from build123d import *

# Parameters (mm, degrees)
BOSS_EXTRUDE1_DEPTH = 5.0165
SKETCH2_W           = 41.021
SKETCH2_H           = 23.876
BOSS_EXTRUDE2_DEPTH = 11.049


with BuildPart() as part:
    # Sketch1 → Boss-Extrude1 (new, symmetric)
    with BuildSketch(Plane(origin=(0, 0, 0), x_dir=(1, 0, 0), z_dir=(0, 1, 0))):
        Polygon((-18.8595, 0), (18.8595, 0), (20.4978, 6.6675), (27.3558, 6.6675), (27.3558, 10.0838), (44.5897, 10.0838), (44.5897, 0.9398), (49.1871, 0.9398), (49.1871, -5.1943), (39.497, -5.1943), (39.497, -18.4404), (-39.497, -18.4404), (-39.497, -5.1943), (-49.1871, -5.1943), (-49.1871, 0.9398), (-44.5897, 0.9398), (-44.5897, 10.0838), (-27.3558, 10.0838), (-27.3558, 6.6675), (-20.4978, 6.6675), align=None)
    extrude(amount=BOSS_EXTRUDE1_DEPTH, both=True)

    # Sketch2 → Boss-Extrude2 (add, symmetric)
    with BuildSketch(Plane(origin=(0, 0, 0), x_dir=(1, 0, 0), z_dir=(0, 1, 0))):
        with Locations((0, -30.3784)):
            Rectangle(SKETCH2_W, SKETCH2_H)
    extrude(amount=BOSS_EXTRUDE2_DEPTH, both=True)


solid = part.part
Can you work these out from the model? Positions are in its coordinate system, mm. A direction names the side the tool comes from. Coordinates: 2 decimals unless noted, no trailing zeros. Write each loop counter-clockwise with the first axis right and the second up, starting at its lowest first coordinate (ties: lowest second). Pieces come first, ordered by that corner, then holes. Notation, with made-up numbers: M 27.25,12 L 63.25,12 A29 cw 63.25,36 Z; hole C 77,-31.75 d8. An arc over 180 degrees is marked long. Use one line per item in the form item = value.
Q1. For faces 1 (the flat face through (0, 0, 0)), 2 (the flat face through (-44.59, 0, -5)), 3 (the flat face through (20.51, 0, 31)), which set-ups out of +Z, -Z, +X, -X, +Y, -Y let a thin tool reach every point of the face, with its end or its side?
Model answer:
face_1 = -Z, +Y, -Y
face_2 = -Z, -X, +Y, -Y
face_3 = +Z, +X, +Y, -Y
Q2. If we section it at B-B (z = -3.5): Write out the boundary of the cut face in (x, y).
Model answer:
outline = M -44.59,-5.02 L -19.72,-5.02 L -19.72,5.02 L -44.59,5.02 Z; M 19.72,-5.02 L 44.59,-5.02 L 44.59,5.02 L 19.72,5.02 Z
Q3. If we section it at D-D (z = 9.5): Write out the boundary of the cut face in (x, y), then the cut area to 3 significant figures.
Model answer:
outline = M -39.5,-5.02 L 39.5,-5.02 L 39.5,5.02 L -39.5,5.02 Z
area = 793 mm^2
Q4. If we section it at C-C (y = -1.75): Write out the boundary of the cut face in (x, z), then the cut area to 3 significant figures.
Model answer:
outline = M -49.19,-0.94 L -44.59,-0.94 L -44.59,-10.08 L -27.36,-10.08 L -27.36,-6.67 L -20.5,-6.67 L -18.86,0 L 18.86,0 L 20.5,-6.67 L 27.36,-6.67 L 27.36,-10.08 L 44.59,-10.08 L 44.59,-0.94 L 49.19,-0.94 L 49.19,5.19 L 39.5,5.19 L 39.5,18.44 L 20.51,18.44 L 20.51,42.32 L -20.51,42.32 L -20.51,18.44 L -39.5,18.44 L -39.5,5.19 L -49.19,5.19 Z
area = 3,000 mm^2
Q5. I need wall thicknesses on line 1 along X through (y, z) = (-1, 39.5); line 2 along Z through (x, y) = (0, 8.75); line 3 along X through (y, z) = (3, 14). Which ranges of each line are inside material? Lowest first, please. Write a range as from..to.
Model answer:
line_1 = -20.51..20.51
line_2 = 18.44..42.32
line_3 = -39.5..39.5
Q6. If we section it at A-A (x = 17.5): Write out the boundary of the cut face in (y, z), then the cut area to 3 significant figures.
Model answer:
outline = M -11.05,18.44 L -5.02,18.44 L -5.02,0 L 5.02,0 L 5.02,18.44 L 11.05,18.44 L 11.05,42.32 L -11.05,42.32 Z
area = 713 mm^2
Q7. For P1, Ø4, axis at y = -7.5, z = 33.5, coming from the -X side; P2, Ø5, axis at y = 0.5, z = 10.5, coming from the -X side; P3, Ø1.5, axis at x = 22, y = -8, coming from the -Z side; P4, Ø2.5, axis at y = 1, z = -5, coming from the -X side, each with a flat end and sliding along its axis, tell me the tip position at first contact or that it passes through.
Model answer:
P1 = -20.51
P2 = -39.5
P3 = through
P4 = -44.59
